```python
from build123d import *

# Parameters (mm, degrees)
SKETCH_FOOT_AND_SUPPORT_SHELF_W = 16
SKETCH_FOOT_AND_SUPPORT_SHELF_H = 8
FOOT_AND_SUPPORT_SHELF_DEPTH    = 5
CLAMP_UPRIGHT_START             = 5
SKETCH_CLAMP_UPRIGHT_W          = 9.2
SKETCH_CLAMP_UPRIGHT_H          = 8
CLAMP_UPRIGHT_DEPTH             = 6.7
CORNER_RETAINING_LIP_START      = 11.7
SKETCH_CORNER_RETAINING_LIP_W   = 12.2
SKETCH_CORNER_RETAINING_LIP_H   = 8
CORNER_RETAINING_LIP_DEPTH      = 2.8
M3_THROUGH_START                = -1
SKETCH_M3_THROUGH_R             = 1.7
M3_THROUGH_DEPTH                = 17


with BuildPart() as part:
    # Sketch_Foot_and_support_shelf → Foot_and_support_shelf (new body)
    with BuildSketch(Plane.XY):
        with Locations((3.5, 0)):
            Rectangle(SKETCH_FOOT_AND_SUPPORT_SHELF_W, SKETCH_FOOT_AND_SUPPORT_SHELF_H)
    extrude(amount=FOOT_AND_SUPPORT_SHELF_DEPTH)

    # Sketch_Clamp_upright → Clamp_upright (add)
    with BuildSketch(Plane.XY.offset(CLAMP_UPRIGHT_START)):
        Rectangle(SKETCH_CLAMP_UPRIGHT_W, SKETCH_CLAMP_UPRIGHT_H)
    extrude(amount=CLAMP_UPRIGHT_DEPTH)

    # Sketch_Corner_retaining_lip → Corner_retaining_lip (add)
    with BuildSketch(Plane.XY.offset(CORNER_RETAINING_LIP_START)):
        with Locations((1.5, 0)):
            Rectangle(SKETCH_CORNER_RETAINING_LIP_W, SKETCH_CORNER_RETAINING_LIP_H)
    extrude(amount=CORNER_RETAINING_LIP_DEPTH)

    # Sketch_M3_through → M3_through (cut)
    with BuildSketch(Plane.XY.offset(M3_THROUGH_START)):
        Circle(SKETCH_M3_THROUGH_R)
    extrude(amount=M3_THROUGH_DEPTH, mode=Mode.SUBTRACT)


solid = part.part
```
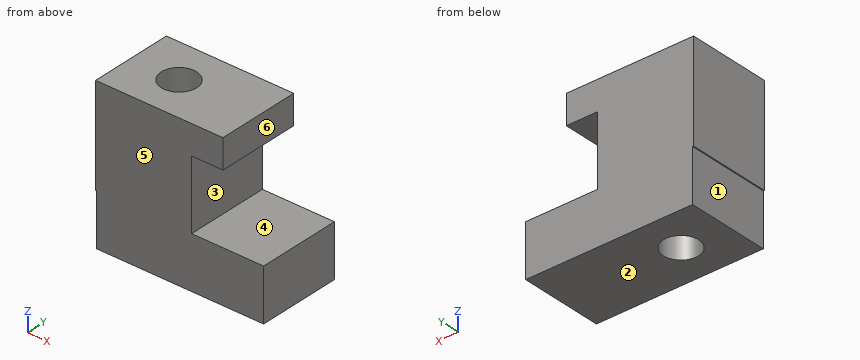
The listing builds one solid part. Answer for the finished solid, in the listing's coordinates (mm). Face numbers are marked on the shaded views. A direction names the side the tool comes from. Coordinates: 2 decimals unless noted, no trailing zeros. Write each loop counter-clockwise with the first axis right and the second up, starting at its lowest first coordinate (ties: lowest second). Pieces come first, ordered by that corner, then holes. Notation, with made-up numbers: (-29.5, 34) -> (11.5, 34) arc R34 cw to (11.5, 70) -> close; hole circle Ø10 at (-35, 85). An arc over 180 degrees is marked (long way). Write each question's results on one line, items separated by ' | '. Start each with the question number.
1) For a pull along Z with two mould halves and no side action, classify the marked faces 1, 2 and 3 as +Z half, -Z half, draft (parallel to the pull), parting line (faces both ways), or undercut.
2) A cutting plane is placed at C-C (z = 9.5). Determine the outline of the cut face in (x, y).
3) Straight lines are drawn through the part: probe 1 along Y at (x, z) = (0, 8.75); probe 2 along Z at (x, y) = (6.75, -3); probe 3 along X at (y, z) = (0, 5.5). For each, find the intervals that lie inside material, in ascending order.
4) Flat-ended cylindrical pins translate along their axes: pin 1 Ø1.5 at (y, z) = (1.5, 2) entering from -X; pin 2 Ø2 at (y, z) = (0, 13.5) entering from +X. Find the tip coordinate at first contact, or state that the pin passes through.
5) A cutting plane is placed at B-B (y = 0). Determine the outline of the cut face in (x, z), then the cut area to 4 significant figures.
6) A cutting plane is placed at A-A (x = 0). Determine the outline of the cut face in (y, z).
7) A tool of negligible diameter and unlimited length cuts with its end or side. For the marked faces 4, 5 and 6, from which of +Z, -Z, +X, -X, +Y, -Y can it reach the whole face along a straight path? Write none if from no direction.
8) A cutting plane is placed at D-D (x = 6). Determine the outline of the cut face in (y, z).
Values follow:
1) face 1: draft | face 2: -Z half | face 3: undercut
2) outline: (-4.6, -4) -> (4.6, -4) -> (4.6, 4) -> (-4.6, 4) -> close; hole circle Ø3.4 at (0, 0)
3) probe 1: -4 to -1.7, 1.7 to 4 | probe 2: 0 to 5, 11.7 to 14.5 | probe 3: -4.6 to -1.7, 1.7 to 4.6
4) pin 1: x = -4.5 | pin 2: x = 7.6
5) outline: (-4.6, 5) -> (-4.5, 5) -> (-4.5, 0) -> (-1.7, 0) -> (-1.7, 14.5) -> (-4.6, 14.5) -> close; (1.7, 0) -> (11.5, 0) -> (11.5, 5) -> (4.6, 5) -> (4.6, 11.7) -> (7.6, 11.7) -> (7.6, 14.5) -> (1.7, 14.5) -> close | area: 126.5 mm²
6) outline: (-4, 0) -> (-1.7, 0) -> (-1.7, 14.5) -> (-4, 14.5) -> close; (1.7, 0) -> (4, 0) -> (4, 14.5) -> (1.7, 14.5) -> close
7) face 4: +X, +Y, -Y | face 5: +Z, -Z, +X, -X, -Y | face 6: +Z, +X, +Y, -Y
8) outline: (-4, 0) -> (4, 0) -> (4, 5) -> (-4, 5) -> close; (-4, 11.7) -> (4, 11.7) -> (4, 14.5) -> (-4, 14.5) -> close
